The listing builds one solid part. Answer for the finished solid, in the listing's coordinates (mm). A direction names the side the tool comes from. Coordinates: 2 decimals unless noted, no trailing zeros. Loops run counter-clockwise (first coordinate to the right, second up) from the corner with the lowest first, then second, coordinate; pieces in that order, holes last. Notation, with made-up numbers: (57, -9.5) - (71, -9.5) arc R12 ccw to (71, 1.5) - close; hole circle Ø8 at (1, 24.5). An arc over 180 degrees is marked (long way). Write each question's results on one line, items separated by ' | '. Start each with the question number.
(1) Find section B-B on x = -23. Determine the outline of the cut face in (y, z), then the cut area to 4 significant figures.
(2) Determine the mould class of faces 4 (the flat face through (-121, -43, 25)), 5 (the flat face through (-14, -115, 15)), 6 (the flat face through (-14, -128, 15)), 7 (the flat face through (-167, -17, 43)) for opening direction Z: released by +Z, released by -Z, zero draft, split by the parting line, or undercut.
(3) Find section D-D on y = -39. Determine the outline of the cut face in (x, z).
(4) For faces 1 (the flat face through (-8, -132, 2)), 2 (the flat face through (-8, -17, 2)), 3 (the flat face through (-113, -75.5, 25)), determine the directions among +Z, -Z, +X, -X, +Y, -Y from which every point of the face is accessible in a straight line to the end or side of a thin tool.
(5) Find section A-A on y = -119.5. Determine the outline of the cut face in (x, z).
(6) Find section C-C on z = 31. Determine the outline of the cut face in (x, y), then the cut area to 3 significant figures.
(7) Given pin 1 Ø0.6 at (y, z) = (-24, 44) entering from -X; pin 2 Ø0.6 at (y, z) = (-29.5, 43.5) entering from +X; pin 3 Ø8 at (x, y) = (-80.5, -110.5) entering from +Z, each flat-ended and moving along its own axis, determine where each tip first touches the part or whether it passes through.
(8) Consider line 1 (X direction, y = -43.5, z = 17.5); line 2 (X direction, y = -139, z = 19); line 3 (Y direction, x = -114, z = 25.5). Determine where each line is inside the solid, lowest interval first. Write a range as from..to.
from build123d import *

# Parameters (mm, degrees)
SKETCH2_W           = 175
SKETCH2_H           = 150
BOSS_EXTRUDE1_DEPTH = 45
CUT_EXTRUDE1_DEPTH  = 40
SKETCH5_W           = 13
SKETCH5_H           = 13
CUT_EXTRUDE3_DEPTH  = 50
SKETCH6_W           = 10
SKETCH6_H           = 53
CUT_EXTRUDE4_DEPTH  = 2
SKETCH7_W           = 35
SKETCH7_H           = 130
CUT_EXTRUDE5_DEPTH  = 40
SKETCH9_W           = 16
SKETCH9_H           = 35
CUT_EXTRUDE6_DEPTH  = 2
SKETCH10_W          = 16.5
SKETCH10_H          = 24.5
CUT_EXTRUDE7_DEPTH  = 40
SKETCH11_W          = 16
SKETCH11_H          = 35
CUT_EXTRUDE8_DEPTH  = 2
FILLET1_R           = 3


with BuildPart() as part:
    # Sketch2 → Boss-Extrude1 (new body)
    with BuildSketch(Plane.XY):
        with Locations((-87.5, -75)):
            Rectangle(SKETCH2_W, SKETCH2_H)
    extrude(amount=BOSS_EXTRUDE1_DEPTH)

    # Sketch3 → Cut-Extrude1 (cut)
    with BuildSketch(Plane.XY.offset(45)):
        Polygon((-104.5, -10), (-29, -10), (-29, -140), (-156, -140), (-156, -100), (-104.5, -100), align=None)
    extrude(amount=-CUT_EXTRUDE1_DEPTH, mode=Mode.SUBTRACT)

    # Sketch5 → Cut-Extrude3 (cut)
    with BuildSketch(Plane(origin=(0, 0, 0), x_dir=(0, 0, -1), z_dir=(1, 0, 0))):
        with Locations((-14.5, -121.5)):
            Rectangle(SKETCH5_W, SKETCH5_H)
    extrude(amount=-CUT_EXTRUDE3_DEPTH, mode=Mode.SUBTRACT)

    # Sketch6 → Cut-Extrude4 (cut)
    with BuildSketch(Plane.XY.offset(45)):
        with Locations((-109.5, -42.5)):
            Rectangle(SKETCH6_W, SKETCH6_H)
        with Locations((-24, -42.5)):
            Rectangle(SKETCH6_W, SKETCH6_H)
    extrude(amount=-CUT_EXTRUDE4_DEPTH, mode=Mode.SUBTRACT)

    # Sketch7 → Cut-Extrude5 (cut)
    with BuildSketch(Plane.XY.offset(45)):
        with Locations((-138.5, -75)):
            Rectangle(SKETCH7_W, SKETCH7_H)
    extrude(amount=-CUT_EXTRUDE5_DEPTH, mode=Mode.SUBTRACT)

    # Sketch9 → Cut-Extrude6 (cut)
    with BuildSketch(Plane.XY.offset(45)):
        with Locations((-167, -17.5)):
            Rectangle(SKETCH9_W, SKETCH9_H)
        with Locations((-167, -132.5)):
            Rectangle(SKETCH9_W, SKETCH9_H)
        with Locations((-8, -132.5)):
            Rectangle(SKETCH9_W, SKETCH9_H)
        with Locations((-8, -17.5)):
            Rectangle(SKETCH9_W, SKETCH9_H)
    extrude(amount=-CUT_EXTRUDE6_DEPTH, mode=Mode.SUBTRACT)

    # Sketch10 → Cut-Extrude7 (cut)
    with BuildSketch(Plane.XY.offset(45)):
        with Locations((-112.75, -87.75)):
            Rectangle(SKETCH10_W, SKETCH10_H)
    extrude(amount=-CUT_EXTRUDE7_DEPTH, mode=Mode.SUBTRACT)

    # Sketch11 → Cut-Extrude8 (cut)
    with BuildSketch(Plane(origin=(0, 0, 0), x_dir=(-1, 0, 0), z_dir=(0, 0, -1))):
        with Locations((8, -17.5)):
            Rectangle(SKETCH11_W, SKETCH11_H)
        with Locations((8, -132.5)):
            Rectangle(SKETCH11_W, SKETCH11_H)
        with Locations((167, -132.5)):
            Rectangle(SKETCH11_W, SKETCH11_H)
        with Locations((167, -17.5)):
            Rectangle(SKETCH11_W, SKETCH11_H)
    extrude(amount=-CUT_EXTRUDE8_DEPTH, mode=Mode.SUBTRACT)

    # Fillet1
    fillet1_edges = [part.edges().sort_by_distance(p)[0] for p in [
        (0, -150, 22.5),
        (-175, -150, 22.5),
        (-175, 0, 22.5),
        (0, 0, 22.5),
    ]]
    fillet(fillet1_edges, radius=FILLET1_R)


solid = part.part
Values:
1) outline: (-150, 0) - (0, 0) - (0, 45) - (-16, 45) - (-16, 43) - (-69, 43) - (-69, 45) - (-150, 45) - close; hole (-128, 8) - (-115, 8) - (-115, 21) - (-128, 21) - close | area: 6,475 mm²
2) face 4: zero draft | face 5: undercut | face 6: undercut | face 7: released by +Z
3) outline: (-175, 0) - (0, 0) - (0, 45) - (-19, 45) - (-19, 43) - (-29, 43) - (-29, 5) - (-104.5, 5) - (-104.5, 43) - (-114.5, 43) - (-114.5, 45) - (-121, 45) - (-121, 5) - (-156, 5) - (-156, 45) - (-175, 45) - close
4) face 1: -Z, +X, -Y | face 2: -Z, +X, +Y | face 3: +Z
5) outline: (-175, 2) - (-159, 2) - (-159, 0) - (-16, 0) - (-16, 2) - (0, 2) - (0, 8) - (-29, 8) - (-29, 5) - (-156, 5) - (-156, 45) - (-159, 45) - (-159, 43) - (-175, 43) - close; (-29, 21) - (0, 21) - (0, 43) - (-16, 43) - (-16, 45) - (-29, 45) - close
6) outline: (-175, -147) arc R3 ccw to (-172, -150) - (-3, -150) arc R3 ccw to (0, -147) - (0, -3) arc R3 ccw to (-3, 0) - (-172, 0) arc R3 ccw to (-175, -3) - close; hole (-156, -140) - (-29, -140) - (-29, -10) - (-104.5, -10) - (-104.5, -75.5) - (-121, -75.5) - (-121, -10) - (-156, -10) - close | area: 10,800 mm²
7) pin 1: stops at x = -159 | pin 2: stops at x = -16 | pin 3: stops at z = 5
8) line 1: x = -175..-156, -121..-104.5, -29..0 | line 2: x = -175..-156, -29..0 | line 3: y = -150..-140, -75.5..0
